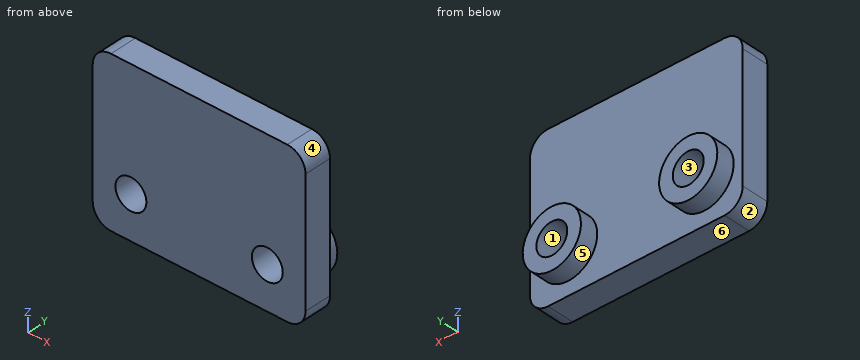
from build123d import *

# Parameters (mm, degrees)
SKETCH_1_W      = 23.4
SKETCH_1_H      = 17.7
SKETCH_1_R      = 1.7
EXTRUDE_1_DEPTH = 3
SKETCH_2_R      = 3.2
SKETCH_2_R_2    = 1.7
EXTRUDE_2_DEPTH = 2
FILLET_1_R      = 2


with BuildPart() as part:
    # Эскиз1 → Бобышка-Вытянуть1 (new body)
    with BuildSketch(Plane(origin=(0, 0, 0), x_dir=(1, 0, 0), z_dir=(0, 1, 0))):
        with Locations((0, -4.15)):
            Rectangle(SKETCH_1_W, SKETCH_1_H)
        with Locations(Location((-7.5, 0, 0), (0, 0, 270))):
            Circle(SKETCH_1_R, mode=Mode.SUBTRACT)
        with Locations(Location((7.5, 0, 0), (0, 0, 90))):
            Circle(SKETCH_1_R, mode=Mode.SUBTRACT)
    extrude(amount=EXTRUDE_1_DEPTH)

    # Эскиз2 → Бобышка-Вытянуть2 (add)
    # profile 1 of 2: a face of its own
    with BuildSketch(Plane(origin=(0, 3, 0), x_dir=(1, 0, 0), z_dir=(0, 1, 0))):
        with Locations(Location((-7.5, 0, 0), (0, 0, 270))):
            Circle(SKETCH_2_R)
        with Locations(Location((-7.5, 0, 0), (0, 0, 270))):
            Circle(SKETCH_2_R_2, mode=Mode.SUBTRACT)
    # profile 2 of 2: a face of its own
    with BuildSketch(Plane(origin=(0, 3, 0), x_dir=(1, 0, 0), z_dir=(0, 1, 0))):
        with Locations(Location((7.5, 0, 0), (0, 0, 270))):
            Circle(SKETCH_2_R)
        with Locations(Location((7.5, 0, 0), (0, 0, 90))):
            Circle(SKETCH_2_R_2, mode=Mode.SUBTRACT)
    extrude(amount=EXTRUDE_2_DEPTH)

    # Скругление1
    fillet_1_edges = [part.edges().sort_by_distance(p)[0] for p in [
        (-11.7, 1.5, -4.7),
        (11.7, 1.5, -4.7),
        (11.7, 1.5, 13),
        (-11.7, 1.5, 13),
    ]]
    fillet(fillet_1_edges, radius=FILLET_1_R)


solid = part.part
Verification items for the finished model (mm, model axes). Face numbers are marked on the shaded views. A direction names the side the tool comes from. Coordinates: 2 decimals unless noted, no trailing zeros. Order: outer loops, then holes, each group sorted by start corner. A loop starts at its lowest first (then second) coordinate and runs counter-clockwise, first axis right, second up. Notation, with made-up numbers: M -11.5,9 L 10.5,9 A7 ccw 10.5,17 Z; hole C 79.25,78.5 d1. An arc over 180 degrees is marked long. One line per item, written item: value. Start each with the question number.
Item 1: Access from +Z, -Z, +X, -X, +Y, -Y to the whole of each face (thin tool, end or side, straight path). Record for the marked faces 5 and 6.
Item 2: Sectioned sample at C-C on y = 2.6. Record the cut outline in (x, z).
Item 3: Sectioned sample at B-B on z = 0. Record the cut outline in (x, y).
Item 4: Sectioned sample at D-D on x = 8. Record the cut outline in (y, z).
Item 5: Mould release check, pull along Z, two halves, no side actions. Record for the marked faces 1, 2, 3 and 4: pulls with the +Z half, pulls with the -Z half, needs draft (parallel to the pull), parting line crosses it, or undercut.
Item 6: Thickness scan on probe 1 along X at (y, z) = (3.1, 0); probe 2 along X at (y, z) = (2.6, 0); probe 3 along X at (y, z) = (4.1, 1). Record the ranges inside material, lowest first.
Item 7: Depth check by flat-ended pin: P1, Ø1, axis at x = -2, z = 5.5, coming from the +Y side; P2, Ø3, axis at y = 3.5, z = 9, coming from the +X side. Enter the tip coordinate at first touch or a pass-through.
Item 8: Sectioned sample at A-A on x = -7.5. Record the cut outline in (y, z).
Calculated:
1. face 5: +Y
1. face 6: -Z, +X, -X, +Y, -Y
2. outline: M -11.7,-2.7 A2 ccw -9.7,-4.7 L 9.7,-4.7 A2 ccw 11.7,-2.7 L 11.7,11 A2 ccw 9.7,13 L -9.7,13 A2 ccw -11.7,11 Z; hole C -7.5,0 d3.4; hole C 7.5,0 d3.4
3. outline: M -11.7,0 L -9.2,0 L -9.2,5 L -10.7,5 L -10.7,3 L -11.7,3 Z; M -5.8,0 L 5.8,0 L 5.8,5 L 4.3,5 L 4.3,3 L -4.3,3 L -4.3,5 L -5.8,5 Z; M 9.2,0 L 11.7,0 L 11.7,3 L 10.7,3 L 10.7,5 L 9.2,5 Z
4. outline: M 0,-4.7 L 3,-4.7 L 3,-3.16 L 5,-3.16 L 5,-1.62 L 0,-1.62 Z; M 0,1.62 L 5,1.62 L 5,3.16 L 3,3.16 L 3,13 L 0,13 Z
5. face 1: undercut
5. face 2: pulls with the -Z half
5. face 3: undercut
5. face 4: pulls with the +Z half
6. probe 1: -10.7 to -9.2, -5.8 to -4.3, 4.3 to 5.8, 9.2 to 10.7
6. probe 2: -11.7 to -9.2, -5.8 to 5.8, 9.2 to 11.7
6. probe 3: -10.54 to -8.87, -6.13 to -4.46, 4.46 to 6.13, 8.87 to 10.54
7. P1: y = 3
7. P2: x = 11.7
8. outline: M 0,-4.7 L 3,-4.7 L 3,-3.2 L 5,-3.2 L 5,-1.7 L 0,-1.7 Z; M 0,1.7 L 5,1.7 L 5,3.2 L 3,3.2 L 3,13 L 0,13 Z
